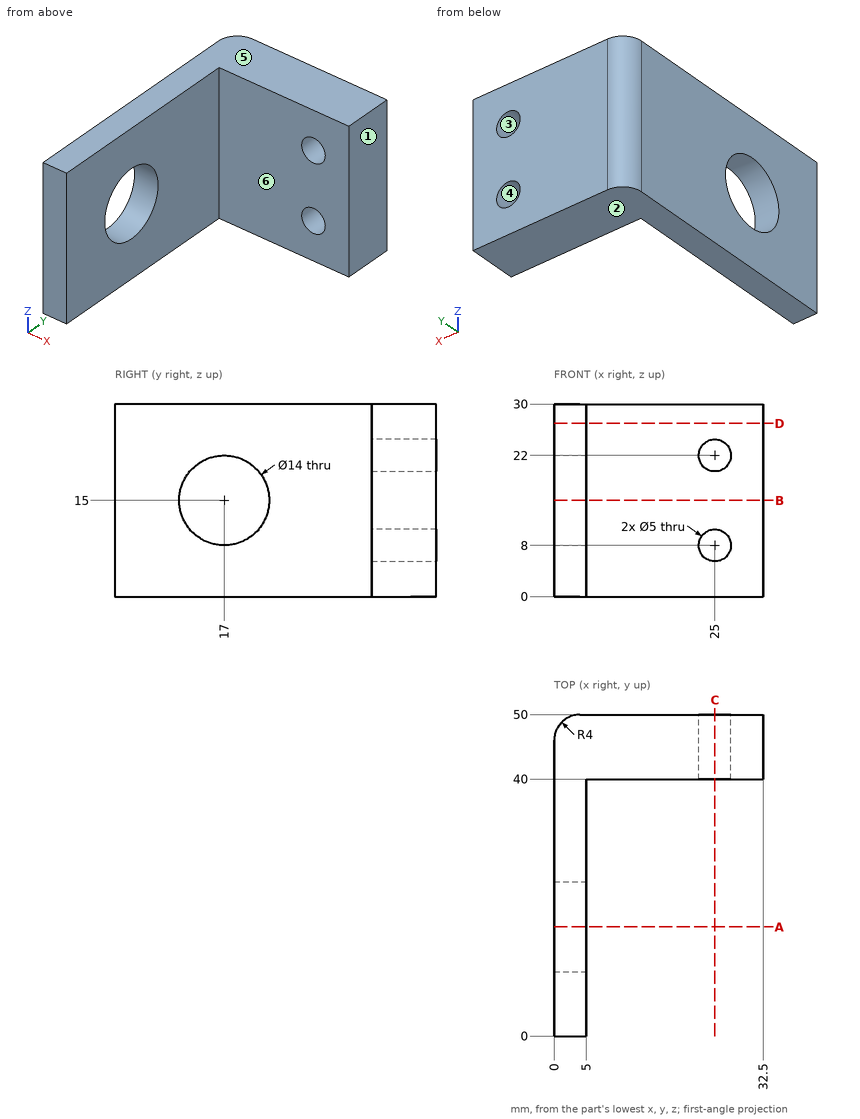
Geometry check sheet. Reference: drawing and pictorial views, mm from the part's lowest x, y, z. A direction names the side the tool comes from. Round coordinates to 2 decimals unless told otherwise and drop trailing zeros. Write each loop counter-clockwise with the first axis right and the second up, starting at its lowest first coordinate (ties: lowest second). Pieces come first, ordered by that corner, then holes. Notation, with made-up numbers: (22.25, 32) -> (34.25, 32) arc R20 cw to (34.25, 51) -> close; hole circle Ø7 at (15, 39). An arc over 180 degrees is marked (long way). Answer as CSV lines item,"result". Start each with the question number.
1) Section check B-B on z = 15. Enter the section's corners in (x, y), and give its area (3 significant figures).
2) Release check for a two-part mould opening along Z. For the marked faces 1, 2, 3 and 4 record: pulls with the +Z half, pulls with the -Z half, needs draft (parallel to the pull), parting line crosses it, or undercut.
3) Material ranges on line 1 (X direction, y = 43, z = 22); line 2 (Y direction, x = 15.5, z = 25.25); line 3 (Y direction, x = 3.5, z = 11.75), recorded low to high. Write a range as from..to.
4) Section check D-D on z = 27. Enter the section's corners in (x, y).
5) Section check C-C on x = 25. Enter the section's corners in (y, z).
6) Section check A-A on y = 17. Enter the section's corners in (x, z), and give its area (3 significant figures).
7) Tool access check on the marked faces 5 and 6. Record the directions out of +Z, -Z, +X, -X, +Y, -Y that give a thin tool (end or side, any length) a straight path to the whole face; none if there is none.
8) Go/stop test with flat-tipped pins: P1, Ø6.5, axis at x = 25, z = 22, coming from the -Y side; P2, Ø16, axis at y = 17, z = 15, coming from the -X side; P3, Ø5, axis at y = 27.5, z = 9.5, coming from the +X side. Record where each tip stops, or that it passes through.
Found:
1,outline,"(0, 0) -> (5, 0) -> (5, 10) -> (0, 10) -> close; (0, 24) -> (5, 24) -> (5, 40) -> (32.5, 40) -> (32.5, 50) -> (4, 50) arc R4 ccw to (0, 46) -> close"
1,area,"452 mm^2"
2,face 1,"needs draft"
2,face 2,"pulls with the -Z half"
2,face 3,"undercut"
2,face 4,"undercut"
3,line 1,"x = 0..22.5, 27.5..32.5"
3,line 2,"y = 40..50"
3,line 3,"y = 0..10.8, 23.2..49.97"
4,outline,"(0, 0) -> (5, 0) -> (5, 40) -> (32.5, 40) -> (32.5, 50) -> (4, 50) arc R4 ccw to (0, 46) -> close"
5,outline,"(40, 0) -> (50, 0) -> (50, 5.5) -> (40, 5.5) -> close; (40, 10.5) -> (50, 10.5) -> (50, 19.5) -> (40, 19.5) -> close; (40, 24.5) -> (50, 24.5) -> (50, 30) -> (40, 30) -> close"
6,outline,"(0, 0) -> (5, 0) -> (5, 8) -> (0, 8) -> close; (0, 22) -> (5, 22) -> (5, 30) -> (0, 30) -> close"
6,area,"80.0 mm^2"
7,face 5,"+Z, +X, -X, +Y, -Y"
7,face 6,"+Z, -Z, +X, -Y"
8,P1,"stops at y = 40"
8,P2,"stops at x = 0"
8,P3,"stops at x = 5"
